Autodesk Inventor part; units mm, degrees
ref_plane "Work Plane1" through (0, 0, -15) normal (0, 0, 1) x (1, 0, 0)
ref_plane "YZ Plane" through (0, 0, 0) normal (1, 0, 0) x (0, 1, 0)
ref_plane "XZ Plane" through (0, 0, 0) normal (0, 1, 0) x (-1, 0, 0)
sketch "Sketch1" plane through (0, 0, 0) normal (0, 0, 1) x (1, 0, 0)
  line L0 (0, 0) -> (25, 0)
  line L1 (25, 0) -> (25, 40)
  line L2 (25, 40) -> (0, 40)
  line L3 (0, 40) -> (0, 0)
  dimension "d1" = 25
  dimension "d2" = 40
  dimension "d3" = 25
extrude "Extrusion1" add sketch "Sketch1" against normal blind 30
sketch "Sketch2" plane through (25, 0, 0) normal (1, 0, 0) x (0, 0, -1)
  line L0 (0, 0) -> (30, 0)
  circle A0 centre (15, 6.56) radius 2.46
extrude "Extrusion2" cut sketch "Sketch2" against normal blind 30
sketch "Sketch3" plane through (0, 0, 0) normal (-1, 0, 0) x (0, 0, 1)
  line L0 (0, 0) -> (-30, 0)
  line L1 (-25.05, 0) -> (-4.95, 0)
  line L2 (-4.95, 0) -> (-4.95, 33.12)
  line L3 (-4.95, 33.12) -> (-25.05, 33.12)
  line L4 (-25.05, 33.12) -> (-25.05, 0)
  dimension "d11" = 20.1
extrude "Extrusion3" cut sketch "Sketch3" against normal blind 20
sketch "Sketch4" plane through (0, 0, 0) normal (0, -1, 0) x (1, 0, 0)
  line L0 (20, -4.95) -> (20, -25.05)
  line L1 (20, -15) -> (25, -15)
  line L2 (25, 0) -> (25, -30)
  line L3 (20, -8.025) -> (25, -8.025)
  line L4 (25, -8.025) -> (25, -21.975)
  line L5 (25, -21.975) -> (20, -21.975)
  line L6 (20, -21.975) -> (20, -8.025)
  line L7 (20, -8.025) -> (25, -21.975) construction
  line L8 (25, -8.025) -> (20, -21.975) construction
  line L9 (25, -12.54) -> (25, -17.46)
  point P0 (0, 0)
  point P1 (22.5, -15)
  dimension "d14" = 13.95
extrude "Extrusion4" add sketch "Sketch4" along normal blind 15
sketch "Sketch5" plane through (20, 0, 0) normal (-1, 0, 0) x (0, 0, 1)
  circle A0 centre (-15, 6.56) radius 2.46
  circle A1 centre (-15, 6.56) radius 4.7025
  circle A2 centre (-15, 6.56) radius 2.46
  circle A3 centre (-15, 6.56) radius 2.46
  point P0 (0, 0)
  dimension "d17" = 9.405
extrude "Extrusion5" cut sketch "Sketch5" against normal blind 2.1
sketch "Sketch6" plane through (25, 0, 0) normal (1, 0, 0) x (0, 0, -1)
  circle A0 centre (15, 6.56) radius 4.7025
  line L0 (15, 6.56) -> (15, 23.56)
  circle A1 centre (15, 23.56) radius 2.46
  point P0 (0, 0)
  dimension "d20" = 17
  dimension "d21" = 4.92
extrude "Extrusion6" cut sketch "Sketch6" against normal blind 10 contours A1
sketch "Sketch7" plane through (20, 0, 0) normal (-1, 0, 0) x (0, 0, 1)
  circle A0 centre (-15, 23.56) radius 2.46
  circle A1 centre (-15, 23.56) radius 4.7025
  point P0 (0, 0)
  dimension "d24" = 9.405
extrude "Extrusion7" cut sketch "Sketch7" against normal blind 2.1
sketch "Sketch9" plane through (25, 0, 0) normal (1, 0, 0) x (0, 0, -1)
  circle A0 centre (15, 6.56) radius 2.46
  circle A1 centre (15, 6.56) radius 2.46
  circle A2 centre (15, 23.56) radius 2.46
  circle A3 centre (15, 23.56) radius 2.46
  line L0 (30, 40) -> (30, 0)
  line L1 (30, 0) -> (30, 40)
  line L2 (30, 40) -> (0, 40)
  line L3 (0, 40) -> (0, 0)
  line L4 (0, 0) -> (8.025, 0)
  line L5 (21.975, 0) -> (21.975, -15)
  line L6 (21.975, -15) -> (8.025, -15)
  line L7 (8.025, -15) -> (8.025, 0)
  line L8 (0, 0) -> (8.025, 0)
  line L9 (21.975, 0) -> (30, 0)
extrude "Extrusion8" add sketch "Sketch9" along normal blind 5
sketch "Sketch10" plane through (0, 40, 0) normal (0, 1, 0) x (1, 0, 0)
  line L0 (0, 30) -> (30, 30)
  line L1 (30, 0) -> (0, 0)
  line L2 (0, 30) -> (30, 30)
  line L3 (30, 30) -> (30, 0)
  line L4 (30, 0) -> (0, 0)
  line L5 (0, 0) -> (0, 30)
extrude "Extrusion9" add sketch "Sketch10" along normal blind 30
sketch "Sketch12" plane through (30, 0, 0) normal (1, 0, 0) x (0, 0, -1)
  circle A0 centre (15, 6.56) radius 2.46
  line L0 (15, 6.56) -> (15, 15.06)
  circle A1 centre (15, 15.06) radius 2.525
  point P0 (0, 0)
  dimension "d31" = 8.5
  dimension "d33" = 5.05
extrude "Extrusion10" cut sketch "Sketch12" against normal blind 30 contours A1
sketch "Sketch15" plane through (0, 0, -25.05) normal (-1, 0, 0) x (0, 0, 1)
  line L0 (0, 33.12) -> (20.1, 33.12)
  line L1 (20.1, 33.12) -> (20.1, 0)
  line L2 (0, 33.12) -> (20.1, 33.12)
  line L3 (20.1, 33.12) -> (20.1, 31.1)
  line L4 (20.1, 31.1) -> (0, 31.1)
  line L5 (0, 31.1) -> (0, 33.12)
  point P0 (25.05, 0)
  dimension "d57" = 2.02
extrude "Extrusion13" add sketch "Sketch15" against normal blind 20
sketch "Sketch17" plane through (0, 0, 0) normal (0, 0, 1) x (1, 0, 0)
  line L0 (0, 70) -> (30, 70)
  line L1 (30, 70) -> (50.0622, 90.0622)
  line L2 (30, 70) -> (80, 70) construction
  line L3 (11.9522, 97.2454) -> (0, 85.2932)
  line L4 (0, 70) -> (0, 85.2932)
  line L5 (0, 70) -> (0, 0)
  line L6 (0, 70) -> (30, 70)
  line L7 (10.923, 112.2849) -> (0, 120.567)
  line L8 (2.5, 134.067) -> (0, 135.567)
  line L9 (2.5, 134.067) -> (5, 128.067)
  line L10 (2.5, 122.067) -> (0, 120.567)
  line L11 (2.5, 122.067) -> (5, 128.067)
  line L12 (50.0622, 105.3553) -> (50.0622, 120.567)
  line L13 (50.0622, 105.3553) -> (50.0622, 90.0622)
  line L14 (0, 135.567) -> (30, 135.567)
  line L15 (30, 135.567) -> (50.0622, 120.567)
  arc A0 (11.9522, 97.2454) -> (10.923, 112.2849) centre (4.8811, 104.3165) ccw
  dimension "d61" = 45
  dimension "d62" = 32.0271
  dimension "d71" = 30
  dimension "d72" = 10
extrude "Extrusion14" add sketch "Sketch17" against normal blind 30
sketch "Sketch19" plane through (0, 0, 0) normal (0, 0, 1) x (1, 0, 0)
  line L0 (30, 0) -> (30, 70)
  line L1 (30, 70) -> (50.0622, 90.0622)
  line L2 (30, 70) -> (50.0622, 90.0622)
  line L3 (50.0622, 120.567) -> (50.0622, 90.0622)
  line L4 (50.0622, 90.0622) -> (50.0622, 120.567)
  line L5 (30, 135.567) -> (50.0622, 120.567)
  line L6 (50.0622, 120.567) -> (30, 135.567)
  line L7 (0, 135.567) -> (30, 135.567)
  line L8 (30, 135.567) -> (0, 135.567)
  line L9 (5, 128.067) -> (2.5, 134.067)
  line L10 (0, 135.567) -> (2.5, 134.067)
  line L11 (2.5, 134.067) -> (5, 128.067)
  line L12 (2.5, 122.067) -> (5, 128.067)
  line L13 (5, 128.067) -> (2.5, 122.067)
  line L14 (0, 120.567) -> (2.5, 122.067)
  line L15 (2.5, 122.067) -> (0, 120.567)
  line L16 (10.923, 112.2849) -> (0, 120.567)
  line L17 (0, 120.567) -> (10.923, 112.2849)
  line L18 (11.9522, 97.2454) -> (0, 85.2932)
  line L19 (11.9522, 97.2454) -> (0, 85.2932)
  line L20 (0, 85.2932) -> (0, 55.2932)
  line L21 (0, 0) -> (0, 85.2932)
  line L22 (0, 55.2932) -> (30, 55.2932)
  line L23 (30, 55.2932) -> (30, 70)
  arc A0 (11.9522, 97.2454) -> (10.923, 112.2849) centre (4.8811, 104.3165) ccw
  dimension "d75" = 30
  dimension "d76" = 30
extrude "Extrusion15" add sketch "Sketch19" along normal blind 15
ref_plane "Work Plane1" through (0, 0, -15) normal (0, 0, 1) x (1, 0, 0)
mirror "Mirror1" about plane through (0, 0, -15) normal (0, 0, 1) of "Extrusion15"
properties part number "rec_c_12mm_x_60mm"
Can you work these out from the model? Positions are in its coordinate system, mm. A direction names the side the tool comes from. Coordinates: 2 decimals unless noted, no trailing zeros. Loops run counter-clockwise (first coordinate to the right, second up) from the corner with the lowest first, then second, coordinate; pieces in that order, holes last. Notation, with made-up numbers: (82.5, 78.25) -> (86.5, 78.25) arc R18 ccw to (86.5, 87.25) -> close; hole circle Ø2 at (43.5, 41). An arc over 180 degrees is marked (long way). Put each result on its own line as item: value. Start each with the question number.
Q1. I want a section at B-B (x = 26.5). Write out the boundary of the cut face in (y, z) (3 decimals).
Q2. I want a section at C-C (z = -3.5). Write out the boundary of the cut face in (x, y), plus the area to 3 significant figures.
Q3. I want a section at A-A (y = 15.06). Write out the boundary of the cut face in (x, z) (3 decimals), plus the area to 4 significant figures.
Q4. For faces 4 (the face through (5.39, 116.48, -14.58)), 5 (the face through (18, 0, -27)), 6 (the face through (22.1, 4.5, -13)), 7 (the face through (15, 55.293, 7)), 8 (the face through (10, 31.1, -15)), which set-ups out of +Z, -Z, +X, -X, +Y, -Y let a thin tool reach every point of the face, with its end or its side?
Q5. Thinking about a two-plate mould opening in Z: for faces 1 (the face through (15, 0, -3)), 2 (the face through (15, 28, 0)), 3 (the face through (20, 8, -20)), which applies, pulls with the +Z half, pulls with the -Z half, needs draft (parallel to the pull), parting line crosses it, or undercut?
Q6. I'm going to push flat-ended pins straight in: P1, Ø5, axis at x = 14, y = 5, coming from the -Z side; P2, Ø12, axis at x = 9, z = 8.5, coming from the -Y side; P3, Ø5.5, axis at y = 6.56, z = -15, coming from the +X side; P4, Ø3, axis at y = 23.56, z = -15, coming from the -X side. Where does each tip first touch, or does it pass through?
Q7. I want a section at D-D (x = 17.5). Write out the boundary of the cut face in (y, z), plus the area to 3 significant figures.
Q8. If I drill on line 1 (Y direction, x = 26.25, z = -15) (3 decimals); line 2 (Z direction, x = 27, y = 15); line 3 (Z direction, x = 21, y = 6), over which ranges is the centre line in solid material (lowest first)? Write a range as [from, to].
Taken from the geometry:
1. outline: (-15, -21.975) -> (0, -21.975) -> (0, -30) -> (55.293, -30) -> (55.293, -45) -> (135.567, -45) -> (135.567, 15) -> (55.293, 15) -> (55.293, 0) -> (0, 0) -> (0, -8.025) -> (-15, -8.025) -> close; hole circle Ø4.92 at (6.56, -15); hole circle Ø5.05 at (15.06, -15); hole circle Ø4.92 at (23.56, -15)
2. outline: (0, 0) -> (30, 0) -> (30, 70) -> (50.06, 90.06) -> (50.06, 120.57) -> (30, 135.57) -> (0, 135.57) -> (2.5, 134.07) -> (5, 128.07) -> (2.5, 122.07) -> (0, 120.57) -> (10.92, 112.28) arc R10 cw to (11.95, 97.25) -> (0, 85.29) -> close
2. area: 4,660 mm2
3. outline: (0, -30) -> (30, -30) -> (30, -17.525) -> (20, -17.525) -> (20, -25.05) -> (0, -25.05) -> close; (0, -4.95) -> (20, -4.95) -> (20, -12.475) -> (30, -12.475) -> (30, 0) -> (0, 0) -> close
3. area: 447.5 mm2
4. face 4: +Z, -Z, -X
4. face 5: -Z, +X, -X, -Y
4. face 6: -X
4. face 7: +Z, +X, -X, -Y
4. face 8: -X, -Y
5. face 1: needs draft
5. face 2: pulls with the +Z half
5. face 3: undercut
6. P1: stops at z = -30
6. P2: stops at y = 55.29
6. P3: stops at x = 30
6. P4: passes through
7. outline: (0, -30) -> (55.29, -30) -> (55.29, -45) -> (135.57, -45) -> (135.57, 15) -> (55.29, 15) -> (55.29, 0) -> (0, 0) -> (0, -4.95) -> (31.1, -4.95) -> (31.1, -25.05) -> (0, -25.05) -> close
7. area: 5,850 mm2
8. line 1: y = [-15, 4.1], [9.02, 12.535], [17.585, 21.1], [26.02, 135.567]
8. line 2: z = [-30, -17.52], [-12.48, 0]
8. line 3: z = [-30, -19.67], [-10.33, 0]
